```python
from build123d import *

# Parameters (mm, degrees)
SKETCH1_W           = 48.5
SKETCH1_H           = 45.5
BOSS_EXTRUDE1_DEPTH = 3
BOSS_EXTRUDE2_DEPTH = 47
SKETCH3_W           = 5
SKETCH3_H           = 40
BOSS_EXTRUDE3_DEPTH = 40
BOSS_EXTRUDE4_DEPTH = 5
FILLET1_R           = 8
SKETCH5_R           = 1.75
SKETCH5_R_2         = 12.5
CUT_EXTRUDE1_DEPTH  = 128.550617748
SKETCH7_R           = 1.75
CUT_EXTRUDE2_DEPTH  = 132.610590713
FILLET2_START       = -21.25
FILLET2_DEPTH       = 13
FILLET2_2_DEPTH     = 5
FILLET2_START_2     = -16.7781
FILLET2_3_DEPTH     = 8.5281
FILLET2_START_3     = -47.0000001
FILLET2_4_DEPTH     = 46.2000001
FILLET3_R           = 5
FILLET4_R           = 2
CHAMFER2_SIZE       = 1.6
FILLET5_R           = 4
FILLET7_R           = 4
FILLET8_R           = 2
CUT_EXTRUDE3_REACH  = 133.064
SKETCH8_W           = 10
SKETCH8_H           = 10
FILLET9_R           = 2
CHAMFER3_SIZE       = 1.6


with BuildPart() as part:
    # Sketch1 → Boss-Extrude1 (new body)
    with BuildSketch(Plane(origin=(0, 0, 0), x_dir=(1, 0, 0), z_dir=(0, 1, 0))):
        with Locations((0, -1.5)):
            Rectangle(SKETCH1_W, SKETCH1_H)
    extrude(amount=BOSS_EXTRUDE1_DEPTH)

    # Sketch2 → Boss-Extrude2 (add)
    with BuildSketch(Plane.XZ):
        Polygon((-21.25, 21.25), (21.25, 21.25), (21.25, -21.25), (24.25, -21.25), (24.25, 24.25), (-24.25, 24.25), (-24.25, -21.25), (-21.25, -21.25), align=None)
    extrude(amount=BOSS_EXTRUDE2_DEPTH)

    # Sketch3 → Boss-Extrude3 (add)
    with BuildSketch(Plane(origin=(24.25, 0, 0), x_dir=(0, 0, -1), z_dir=(1, 0, 0))):
        with Locations((18.75, -30.8)):
            Rectangle(SKETCH3_W, SKETCH3_H)
    extrude(amount=BOSS_EXTRUDE3_DEPTH)

    # Sketch4 → Boss-Extrude4 (add)
    with BuildSketch(Plane(origin=(0, 0, -21.25), x_dir=(-1, 0, 0), z_dir=(0, 0, -1))):
        Polygon((24.25, -10.8), (80.818542495, -67.368542495), (52.534271247, -95.652813742), (24.25, -67.368542495), align=None)
    extrude(amount=-BOSS_EXTRUDE4_DEPTH)

    # Fillet1
    fillet1_edges = [part.edges().sort_by_distance(p)[0] for p in [
        (24.25, -28.9, -16.25),
        (-24.25, -28.9, -16.25),
    ]]
    fillet(fillet1_edges, radius=FILLET1_R)

    # Sketch5 → Cut-Extrude1 (cut, through all)
    with BuildSketch(Plane.XZ):
        with Locations(Location((-15.5, 15.5, 0), (0, 0, 270))):
            Circle(SKETCH5_R)
        with Locations(Location((15.5, 15.5, 0), (0, 0, 270))):
            Circle(SKETCH5_R)
        with Locations(Location((15.5, -15.5, 0), (0, 0, 270))):
            Circle(SKETCH5_R)
        with Locations(Location((-15.5, -15.5, 0), (0, 0, 270))):
            Circle(SKETCH5_R)
        with Locations(Location((0, 0, 0), (0, 0, 270))):
            Circle(SKETCH5_R_2)
    extrude(amount=-CUT_EXTRUDE1_DEPTH, mode=Mode.SUBTRACT)

    # Sketch7 → Cut-Extrude2 (cut, through all)
    with BuildSketch(Plane.XY.offset(-16.25)):
        with Locations((54.25, -20.8)):
            Circle(SKETCH7_R)
        with Locations((54.25, -40.8)):
            Circle(SKETCH7_R)
        with Locations((-66.676406871, -67.368542495)):
            Circle(SKETCH7_R)
        with Locations((-52.534271247, -81.510678119)):
            Circle(SKETCH7_R)
        with Locations((-45.463203436, -46.155339059)):
            Circle(SKETCH7_R)
        with Locations((-31.321067812, -60.297474683)):
            Circle(SKETCH7_R)
        with Locations((39.25, -20.8)):
            Circle(SKETCH7_R)
        with Locations((39.25, -40.8)):
            Circle(SKETCH7_R)
    extrude(amount=-CUT_EXTRUDE2_DEPTH, mode=Mode.SUBTRACT)

    # Fillet2: read off the stored shape, not the designer's step
    # Fillet2 outline → Fillet2 (add)
    with BuildSketch(Plane.XY.offset(FILLET2_START)):
        with BuildLine():
            Line((24.25, -10.8), (34.25, -10.8))
            ThreePointArc((34.25, -10.8), (27.178932188, -7.871067812), (24.25, -0.8))
            Line((24.25, -0.8), (24.25, -10.8))
        make_face()
    extrude(amount=FILLET2_DEPTH)

    # Fillet2 2 outline → Fillet2 2 (add)
    with BuildSketch(Plane.XY.offset(FILLET2_START)):
        with BuildLine():
            Line((-27.178932188, -13.728932188), (-24.25, -10.8))
            Line((-24.25, -10.8), (-24.25, -6.657864376))
            ThreePointArc((-24.25, -6.657864376), (-25.011204675, -10.4846987), (-27.178932188, -13.728932188))
        make_face()
        with BuildLine():
            ThreePointArc((-24.25, -54.141428429), (-23.469544457, -50.268445083), (-21.25, -47))
            Line((-21.25, -47), (-24.25, -47))
            Line((-24.25, -47), (-24.25, -54.141428429))
        make_face()
    extrude(amount=FILLET2_2_DEPTH)

    # Fillet2 3 outline → Fillet2 3 (add)
    with BuildSketch(Plane.XY.offset(FILLET2_START_2)):
        with BuildLine():
            Line((-27.178932188, -13.728932188), (-24.25, -10.8))
            Line((-24.25, -10.8), (-24.25, -6.657864376))
            ThreePointArc((-24.25, -6.657864376), (-25.011204675, -10.4846987), (-27.178932188, -13.728932188))
        make_face()
    extrude(amount=FILLET2_3_DEPTH)

    # Fillet2 4 outline → Fillet2 4 (cut)
    with BuildSketch(Plane(origin=(0, 0, 0), x_dir=(1, 0, 0), z_dir=(0, 1, 0)).offset(FILLET2_START_3)):
        with BuildLine():
            Line((36, 16.250000001), (32.25, 16.25))
            ThreePointArc((32.25, 16.25), (26.593145751, 13.906854249), (24.25, 8.25))
            Line((24.25, 8.25), (36, 8.25))
            Line((36, 8.25), (36, 16.250000001))
        make_face()
        with BuildLine():
            ThreePointArc((-24.25, 8.25), (-25.541796068, 12.608898943), (-29, 15.560095758))
            Line((-29, 15.560095758), (-29, 8.25))
            Line((-29, 8.25), (-24.25, 8.25))
        make_face()
    extrude(amount=FILLET2_4_DEPTH, mode=Mode.SUBTRACT)

    # Fillet3
    fillet3_edges = [part.edges().sort_by_distance(p)[0] for p in [
        (64.25, -10.8, -18.75),
        (64.25, -50.8, -18.75),
        (-24.25, -67.368542495, -18.75),
        (-80.818542495, -67.368542495, -18.75),
        (-52.534271247, -95.652813742, -18.75),
    ]]
    fillet(fillet3_edges, radius=FILLET3_R)

    # Fillet4
    fillet4_edges = [part.edges().sort_by_distance(p)[0] for p in [
        (-21.25, -23.5, 21.25),
        (21.25, -23.5, 21.25),
    ]]
    fillet(fillet4_edges, radius=FILLET4_R)

    # Chamfer2
    chamfer2_edges = [part.edges().sort_by_distance(p)[0] for p in [
        (-15.5, 3, -13.75),
        (15.5, 3, -13.75),
        (15.5, 3, 17.25),
        (-15.5, 3, 17.25),
    ]]
    chamfer(chamfer2_edges, length=CHAMFER2_SIZE)

    # Fillet5
    # the kernel refuses this fillet: 4 mm, written as the material it takes off along each edge
    with BuildSketch(Plane(origin=(24.25, -50.8, -6.262507822), x_dir=(1, 0, 0), z_dir=(0, 0, -1))) as fillet5_piece_1:
        with BuildLine():
            CenterArc((3.994996871, -4), FILLET5_R, 90, 87.134016017)
            Line((0, -3.8), (-0.079899937, -3.796))
            ThreePointArc((-0.079899937, -3.796), (-0.08, -1.9), (-0.08, 0))
            Line((-0.08, 0), (0, 0.08))
            Line((0, 0.08), (3.994996871, 0.08))
            Line((3.994996871, 0.08), (3.994996871, 0))
        make_face()
    extrude(amount=24.974984355, mode=Mode.SUBTRACT)

    # Fillet7
    fillet7_edges = [part.edges().sort_by_distance(p)[0] for p in [
        (24.25, -22, 24.25),
        (-24.25, -22, 24.25),
    ]]
    fillet(fillet7_edges, radius=FILLET7_R)

    # Fillet8
    fillet8_edges = [part.edges().sort_by_distance(p)[0] for p in [
        (24.25, 3, -0.5),
        (0, 3, 24.25),
        (-23.078427125, 3, 23.078427125),
        (23.078427125, 3, 23.078427125),
        (-24.25, 3, -0.5),
    ]]
    fillet(fillet8_edges, radius=FILLET8_R)

    # Sketch8 → Cut-Extrude3 (cut, up to next)
    with BuildSketch(Plane.ZY.offset(24.25), mode=Mode.PRIVATE) as cut_extrude3_sk1:
        with Locations((0, -42)):
            Rectangle(SKETCH8_W, SKETCH8_H)
    cut_extrude3_tool1 = extrude(cut_extrude3_sk1.sketch, amount=-CUT_EXTRUDE3_REACH, mode=Mode.PRIVATE) & part.part
    add(cut_extrude3_tool1.solids().sort_by_distance((-24.25, -42, 0))[0], mode=Mode.SUBTRACT)

    # Fillet9
    fillet9_edges = [part.edges().sort_by_distance(p)[0] for p in [
        (-22.75, -47, -5),
        (-22.75, -37, -5),
        (-22.75, -37, 5),
        (-22.75, -47, 5),
    ]]
    fillet(fillet9_edges, radius=FILLET9_R)

    # Chamfer3
    chamfer3_edges = [part.edges().sort_by_distance(p)[0] for p in [
        (-54.284271247, -81.510678119, -16.25),
        (-47.213203436, -46.155339059, -16.25),
        (-68.426406871, -67.368542495, -16.25),
        (52.5, -40.8, -16.25),
        (37.5, -40.8, -16.25),
        (37.5, -20.8, -16.25),
        (-33.071067812, -60.297474683, -16.25),
        (52.5, -20.8, -16.25),
    ]]
    chamfer(chamfer3_edges, length=CHAMFER3_SIZE)


solid = part.part
```
Verification items for the finished model (mm, model axes). A direction names the side the tool comes from. Give positions to 0.01 mm unless a question says otherwise; leave off trailing zeros. Loops run counter-clockwise (first coordinate to the right, second up) from the corner with the lowest first, then second, coordinate; pieces in that order, holes last.
1. Go/stop test with flat-tipped pins: pin 1 Ø3 at (x, z) = (-11, 18) entering from -Y; pin 2 Ø12.5 at (y, z) = (-14, -9.5) entering from -X; pin 3 Ø2.5 at (x, z) = (48, -19) entering from -Y; pin 4 Ø12 at (x, y) = (25, -15) entering from +Z. Record where each tip stops, or that it passes through.
2. Set-up check for faces 1 (the flat face through (9, 0, 9)), 2 (the flat face through (-23, -42, -5)), 3 (the flat face through (64.25, -31, -19)): record each of +Z, -Z, +X, -X, +Y, -Y from which the full face is reachable in a straight line by a thin tool's end or side.
3. Mould release check, pull along Y, two halves, no side actions. Record for faces 4 (the flat face through (21.25, -23, -1)), 5 (the cylindrical face through (-65.06, -68.04, -19.53)), 6 (the cylindrical face through (-32.71, -61.36, -19.53)), 7 (the flat face through (-66.825, -81.362, -18.785)): released by +Y, released by -Y, zero draft, split by the parting line, or undercut.
4. Section check D-D, the plane x = 0. Enter the section's corners in (y, z), then the cut area to 3 significant figures.
5. Thickness scan on line 1 (Y direction, x = 54.25, z = -18.55); line 2 (X direction, y = -24.5, z = 17); line 3 (X direction, y = -40, z = -19). Record the ranges inside material, lowest first.
6. Section check A-A, the plane x = 39.25. Enter the section's corners in (y, z).
7. Section check C-C, the plane y = -20.8. Count the separate pieces of the cut face and the enclosed holes in it, then the cut area to 3 significant figures.
8. Section check B-B, the plane z = 15.5. Enter the section's corners in (x, y).
Geometry says:
1. pin 1: stops at y = 0
1. pin 2: stops at x = -28.99
1. pin 3: stops at y = -50.8
1. pin 4: stops at z = 24.25
2. face 1: -Z, -Y
2. face 2: -X, -Y
2. face 3: +Z, -Z, +X, +Y, -Y
3. face 4: zero draft
3. face 5: undercut
3. face 6: undercut
3. face 7: released by -Y
4. outline: (-47, 21.25) - (0, 21.25) - (0, 12.5) - (3, 12.5) - (3, 22.25) arc R2 ccw to (1, 24.25) - (-47, 24.25) - close; (0, -21.25) - (3, -21.25) - (3, -12.5) - (0, -12.5) - close
4. area: 202 mm2
5. line 1: y = -50.8 to -42.55, -39.05 to -22.55, -19.05 to -10.8
5. line 2: x = -24.25 to -21.25, 21.25 to 24.25
5. line 3: x = -53.45 to -21.25, 21.25 to 37.69, 40.81 to 52.69, 55.81 to 64.25
6. outline: (-50.8, -21.25) - (-42.55, -21.25) - (-42.55, -17.85) - (-44.15, -16.25) - (-50.8, -16.25) - close; (-39.05, -21.25) - (-22.55, -21.25) - (-22.55, -17.85) - (-24.15, -16.25) - (-37.45, -16.25) - (-39.05, -17.85) - close; (-19.05, -21.25) - (-10.8, -21.25) - (-10.8, -16.25) - (-17.45, -16.25) - (-19.05, -17.85) - close
7. separate pieces: 3
7. enclosed holes: 0
7. area: 633 mm2
8. outline: (-24.25, -47) - (-21.25, -47) - (-21.25, 0) - (-17.25, 0) - (-17.25, 1.4) - (-18.85, 3) - (-22.25, 3) arc R2 ccw to (-24.25, 1) - close; (-13.75, 0) - (13.75, 0) - (13.75, 1.4) - (12.15, 3) - (-12.15, 3) - (-13.75, 1.4) - close; (17.25, 0) - (21.25, 0) - (21.25, -47) - (24.25, -47) - (24.25, 1) arc R2 ccw to (22.25, 3) - (18.85, 3) - (17.25, 1.4) - close
